Read the model definition and answer for the solid it produces. Units are mm, in the model's axes. Face numbers are marked on the shaded views. A direction names the side the tool comes from. Coordinates: 2 decimals unless noted, no trailing zeros. Order: outer loops, then holes, each group sorted by start corner. A loop starts at its lowest first (then second) coordinate and runs counter-clockwise, first axis right, second up. Notation, with made-up numbers: (5.5, 37.25) -> (37.5, 37.25) arc R34 cw to (37.5, 69.25) -> close; hole circle Ø11 at (38.25, 24.5). An arc over 180 degrees is marked (long way). Answer as a JSON object with one key per item and string values. Group by question number.
1) Section A-A on x = -17 is taken. Determine the outline of the cut face in (y, z) (3 decimals), and give its area (3 significant figures).
2) Section B-B on y = 16 is taken. Determine the outline of the cut face in (x, z) (3 decimals), and give its area (3 significant figures).
3) Section D-D on y = 10 is taken. Count the separate pieces of the cut face and the enclosed holes in it, and give its area (3 significant figures).
4) A tool of negligible diameter and unlimited length cuts with its end or side. For the marked faces 5 and 6, from which of +Z, -Z, +X, -X, +Y, -Y can it reach the whole face along a straight path? Write none if from no direction.
5) Section C-C on z = 10 is taken. Determine the outline of the cut face in (x, y) (3 decimals).
6) Consider L1, parallel to Z at x = 17, y = 14 (3 decimals); L2, parallel to Z at x = 52, y = 17.5 (3 decimals); L3, parallel to X at y = 10.75, z = 28 (3 decimals). Determine where each line is inside the solid, lowest interval first.
7) Determine the mould class of the marked faces 1, 2, 3 and 4 for opening direction Z: released by +Z, released by -Z, zero draft, split by the parting line, or undercut.
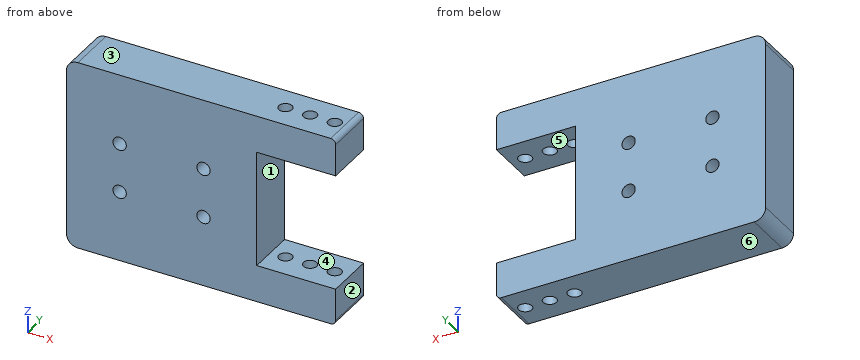
Autodesk Inventor part; units mm, degrees
ref_plane "YZ Plane" through (0, 0, 0) normal (1, 0, 0) x (0, 1, 0)
ref_plane "XZ Plane" through (0, 0, 0) normal (0, 1, 0) x (-1, 0, 0)
ref_plane "XY Plane" through (0, 0, 0) normal (0, 0, 1) x (1, 0, 0)
sketch "Boceto1" plane through (0, 0, 0) normal (0, 1, 0) x (-1, 0, 0)
  line L0 (-38.575, 38.575) -> (38.575, 38.575)
  line L1 (38.575, 38.575) -> (38.575, -38.575)
  line L2 (38.575, -38.575) -> (-38.575, -38.575)
  line L3 (-38.575, -38.575) -> (-38.575, 38.575)
  line L4 (-38.575, 38.575) -> (38.575, -38.575) construction
  line L5 (38.575, 38.575) -> (-38.575, -38.575) construction
  circle A0 centre (17, 10) radius 2.7
  circle A1 centre (17, -10) radius 2.7
  circle A2 centre (-17, -10) radius 2.7
  circle A3 centre (-17, 10) radius 2.7
  point P0 (0, 0)
  dimension "d0" = 77.15
  dimension "d1" = 77.15
  dimension "d2" = 5.4
  dimension "d3" = 10
  dimension "d4" = 10
  dimension "d5" = 17
  dimension "d6" = 17
extrude "Extrusión1" add sketch "Boceto1" along normal blind 20
sketch "Boceto2" plane through (0, 20, 0) normal (0, 1, 0) x (1, 0, 0)
  line L0 (-38.575, -38.575) -> (38.575, -38.575)
  line L1 (38.575, -38.575) -> (70.575, -38.575)
  line L2 (70.575, -38.575) -> (70.575, -23.575)
  line L3 (70.575, -23.575) -> (38.575, -23.575)
  line L4 (38.575, -23.575) -> (38.575, -38.575)
  line L5 (38.575, 38.575) -> (-38.575, 38.575)
  line L6 (38.575, 38.575) -> (70.575, 38.575)
  line L7 (70.575, 38.575) -> (70.575, 23.575)
  line L8 (70.575, 23.575) -> (38.575, 23.575)
  line L9 (38.575, 23.575) -> (38.575, 38.575)
  point P0 (0, 0)
  dimension "d9" = 32
  dimension "d10" = 15
extrude "Extrusión2" add sketch "Boceto2" against normal up to surface (20 mm away)
sketch "Boceto3" plane through (-38.575, 0, 38.575) normal (0, 0, 1) x (1, 0, 0)
  circle A0 centre (103.15, 10) radius 2.7
  circle A1 centre (93.15, 10) radius 2.7
  line L0 (109.15, 20) -> (109.15, 0)
  circle A2 centre (83.15, 10) radius 2.7
  point P0 (38.575, 0)
  dimension "d13" = 5.4
  dimension "d14" = 6
  dimension "d15" = 10
  dimension "d34" = 10
extrude "Extrusión3" cut sketch "Boceto3" against normal through all
fillet "Empalme2" radius 4.635 2 edges at (-38.575, 10, 38.575) (-38.575, 10, -38.575)
fillet "Empalme3" radius 2 2 edges at (70.575, 10, -38.575) (70.575, 10, 38.575)
sketch "Boceto4" plane through (0, 20, 0) normal (0, 1, 0) x (1, 0, 0)
  line L0 (53.225, -32.695) -> (61.325, -32.695)
  line L1 (61.325, -32.695) -> (61.325, -28.455)
  line L2 (61.325, -28.455) -> (53.225, -28.455)
  line L3 (53.225, -28.455) -> (53.225, -32.695)
  line L4 (53.225, -32.695) -> (61.325, -28.455) construction
  line L5 (61.325, -32.695) -> (53.225, -28.455) construction
  line L6 (57.275, -38.575) -> (51.875, -38.575)
  point P0 (0, 0)
  point P1 (57.275, -30.575)
  dimension "d21" = 8.1
  dimension "d23" = 1.35
  dimension "d24" = 8
  dimension "d25" = 4.24
properties part number "UpperJaw" material "Plástico ABS"
Worked answers:
{
 "1": {"outline": "(0, -38.575) -> (20, -38.575) -> (20, -12.7) -> (0, -12.7) -> close; (0, -7.3) -> (20, -7.3) -> (20, 7.3) -> (0, 7.3) -> close; (0, 12.7) -> (20, 12.7) -> (20, 38.575) -> (0, 38.575) -> close", "area": "1,330 mm²"},
 "2": {"outline": "(-38.575, -33.94) arc R4.635 ccw to (-33.94, -38.575) -> (68.575, -38.575) arc R2 ccw to (70.575, -36.575) -> (70.575, -23.575) -> (38.575, -23.575) -> (38.575, 23.575) -> (70.575, 23.575) -> (70.575, 36.575) arc R2 ccw to (68.575, 38.575) -> (-33.94, 38.575) arc R4.635 ccw to (-38.575, 33.94) -> close; hole circle Ø5.4 at (-17, -10); hole circle Ø5.4 at (-17, 10); hole circle Ø5.4 at (17, -10); hole circle Ø5.4 at (17, 10)", "area": "6,810 mm²"},
 "3": {"separate pieces": "7", "enclosed holes": "4", "area": "6,320 mm²"},
 "4": {"face 5": "+X, +Y, -Y", "face 6": "-Z, +X, -X, +Y, -Y"},
 "5": {"outline": "(-38.575, 0) -> (-19.7, 0) -> (-19.7, 20) -> (-38.575, 20) -> close; (-14.3, 0) -> (14.3, 0) -> (14.3, 20) -> (-14.3, 20) -> close; (19.7, 0) -> (38.575, 0) -> (38.575, 20) -> (19.7, 20) -> close"},
 "6": {"L1": "z = -38.575 to -12.7, -7.3 to 7.3, 12.7 to 38.575", "L2": "z = -38.575 to -23.575, 23.575 to 38.575", "L3": "x = -38.575 to 41.981, 47.169 to 51.981, 57.169 to 61.981, 67.169 to 70.575"},
 "7": {"face 1": "undercut", "face 2": "zero draft", "face 3": "released by +Z", "face 4": "undercut"}
}
